Work out the finished part from the listing and answer in its coordinate system (mm). Face numbers are marked on the shaded views. A direction names the side the tool comes from. Give positions to 0.01 mm unless a question says otherwise; leave off trailing zeros. Loops run counter-clockwise (first coordinate to the right, second up) from the corner with the lowest first, then second, coordinate; pieces in that order, holes last. Notation, with made-up numbers: (0, 26.25) - (40, 26.25) arc R31 cw to (40, 55.25) - close; hole circle Ø4 at (27, -17). An arc over 180 degrees is marked (long way). One line per item, written item: value.
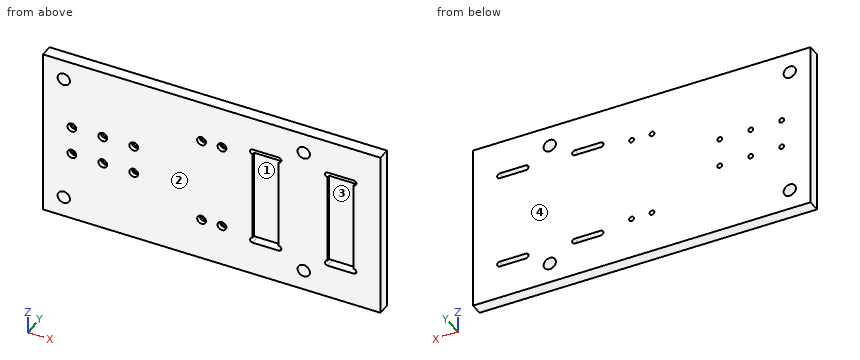
from build123d import *

# Parameters (mm, degrees)
SKETCH1_W                                      = 304.8
SKETCH1_H                                      = 152.4
BOSS_EXTRUDE1_DEPTH                            = 11.1125
CUT_EXTRUDE2_DEPTH                             = 11.1125
SKETCH10_R                                     = 5.55625
CUT_EXTRUDE9_DEPTH                             = 12.1125
CBORE_FOR_8_SOCKET_HEAD_CAP_SCREW1_D           = 4.3053
CBORE_FOR_8_SOCKET_HEAD_CAP_SCREW1_DEPTH       = 11.1125
CBORE_FOR_8_SOCKET_HEAD_CAP_SCREW1_CBORE_D     = 7.9375
CBORE_FOR_8_SOCKET_HEAD_CAP_SCREW1_CBORE_DEPTH = 4.1656
CBORE_FOR_8_SOCKET_HEAD_CAP_SCREW2_D           = 4.3053
CBORE_FOR_8_SOCKET_HEAD_CAP_SCREW2_DEPTH       = 11.1125
CBORE_FOR_8_SOCKET_HEAD_CAP_SCREW2_CBORE_D     = 7.9375
CBORE_FOR_8_SOCKET_HEAD_CAP_SCREW2_CBORE_DEPTH = 4.1656
CUT_EXTRUDE10_REACH                            = 119.196
SKETCH22_W                                     = 23.527686488
SKETCH22_H                                     = 2.54
SKETCH22_W_2                                   = 23.436556581


with BuildPart() as part:
    # Sketch1 → Boss-Extrude1 (new body)
    with BuildSketch(Plane(origin=(0, 0, 0), x_dir=(1, 0, 0), z_dir=(0, 1, 0))):
        with Locations((152.4, 76.2)):
            Rectangle(SKETCH1_W, SKETCH1_H)
    extrude(amount=BOSS_EXTRUDE1_DEPTH)

    # Sketch3 → Cut-Extrude2 (cut)
    with BuildSketch(Plane(origin=(0, 11.1125, 0), x_dir=(1, 0, 0), z_dir=(0, 1, 0))):
        with BuildLine():
            Line((280.567699438, 35.204123045), (257.04001295, 35.204123045))
            ThreePointArc((257.04001295, 35.204123045), (254.65876295, 32.822873045), (257.04001295, 30.441623045))
            Line((257.04001295, 30.441623045), (280.567699438, 30.441623045))
            ThreePointArc((280.567699438, 30.441623045), (282.948949438, 32.822873045), (280.567699438, 35.204123045))
        make_face()
        with BuildLine():
            Line((257.04001295, 117.195876955), (280.567699438, 117.195876955))
            ThreePointArc((280.567699438, 117.195876955), (282.948949438, 119.577126955), (280.567699438, 121.958376955))
            Line((280.567699438, 121.958376955), (257.04001295, 121.958376955))
            ThreePointArc((257.04001295, 121.958376955), (254.65876295, 119.577126955), (257.04001295, 117.195876955))
        make_face()
        with BuildLine():
            Line((212.85998705, 121.958376955), (189.332300562, 121.958376955))
            ThreePointArc((189.332300562, 121.958376955), (186.951050562, 119.577126955), (189.332300562, 117.195876955))
            Line((189.332300562, 117.195876955), (212.85998705, 117.195876955))
            ThreePointArc((212.85998705, 117.195876955), (215.24123705, 119.577126955), (212.85998705, 121.958376955))
        make_face()
        with BuildLine():
            Line((212.85998705, 35.204123045), (189.332300562, 35.204123045))
            ThreePointArc((189.332300562, 35.204123045), (186.951050562, 32.822873045), (189.332300562, 30.441623045))
            Line((189.332300562, 30.441623045), (212.85998705, 30.441623045))
            ThreePointArc((212.85998705, 30.441623045), (215.24123705, 32.822873045), (212.85998705, 35.204123045))
        make_face()
    extrude(amount=-CUT_EXTRUDE2_DEPTH, mode=Mode.SUBTRACT)

    # Sketch10 → Cut-Extrude9 (cut, through all)
    with BuildSketch(Plane.XZ):
        with Locations((18.74955505, -134.149424539)):
            Circle(SKETCH10_R)
        with Locations((18.74955505, -18.250575461)):
            Circle(SKETCH10_R)
        with Locations((235.448687079, -134.149424539)):
            Circle(SKETCH10_R)
        with Locations((235.448687079, -18.250575461)):
            Circle(SKETCH10_R)
    extrude(amount=-CUT_EXTRUDE9_DEPTH, mode=Mode.SUBTRACT)

    # CBORE for #8 Socket Head Cap Screw1
    with Locations(Plane(origin=(143.1925, 0, -37.545187713), x_dir=(0, 0, -1), z_dir=(0, -1, 0))):
        with Locations((0, 0), (0, 18.415), (77.309624574, 18.415), (77.309624574, 0)):
            CounterBoreHole(CBORE_FOR_8_SOCKET_HEAD_CAP_SCREW1_D / 2, CBORE_FOR_8_SOCKET_HEAD_CAP_SCREW1_CBORE_D / 2, CBORE_FOR_8_SOCKET_HEAD_CAP_SCREW1_CBORE_DEPTH, depth=CBORE_FOR_8_SOCKET_HEAD_CAP_SCREW1_DEPTH)

    # CBORE for #8 Socket Head Cap Screw2
    with Locations(Plane(origin=(26.061945565, 0, -89.133574987), x_dir=(0, 0, -1), z_dir=(0, -1, 0))):
        with Locations((0, 0), (-25.867149974, 0), (-25.867149974, 27.94), (0, 27.94), (0, 55.88), (-25.867149974, 55.88)):
            CounterBoreHole(CBORE_FOR_8_SOCKET_HEAD_CAP_SCREW2_D / 2, CBORE_FOR_8_SOCKET_HEAD_CAP_SCREW2_CBORE_D / 2, CBORE_FOR_8_SOCKET_HEAD_CAP_SCREW2_CBORE_DEPTH, depth=CBORE_FOR_8_SOCKET_HEAD_CAP_SCREW2_DEPTH)

    # Sketch22 → Cut-Extrude10 (cut, up to next)
    with BuildSketch(Plane.XY.offset(-35.204123045), mode=Mode.PRIVATE) as cut_extrude10_sk1:
        with Locations((201.096143806, 1.27)):
            Rectangle(SKETCH22_W, SKETCH22_H)
    cut_extrude10_tool1 = extrude(cut_extrude10_sk1.sketch, amount=-CUT_EXTRUDE10_REACH, mode=Mode.PRIVATE) & part.part
    add(cut_extrude10_tool1.solids().sort_by_distance((201.096144, 1.27, -35.204123))[0], mode=Mode.SUBTRACT)
    # Sketch22 → Cut-Extrude10 (cut, up to next)
    with BuildSketch(Plane.XY.offset(-35.204123045), mode=Mode.PRIVATE) as cut_extrude10_sk2:
        with Locations((268.758291241, 1.27)):
            Rectangle(SKETCH22_W_2, SKETCH22_H)
    cut_extrude10_tool2 = extrude(cut_extrude10_sk2.sketch, amount=-CUT_EXTRUDE10_REACH, mode=Mode.PRIVATE) & part.part
    add(cut_extrude10_tool2.solids().sort_by_distance((268.758291, 1.27, -35.204123))[0], mode=Mode.SUBTRACT)


solid = part.part
1. Section C-C (y = 9) is taken. Count the separate pieces of the cut face and the enclosed holes in it, and give its area (3 significant figures).
Output:
separate pieces: 1
enclosed holes: 18
area: 45,400 mm²
2. The mould has two halves that part along Z. Classify the marked faces 1 and 2: released by +Z, released by -Z, zero draft, split by the parting line, or undercut.
Output:
face 1: undercut
face 2: zero draft
3. Section A-A (x = 209.5) is taken. Write down the section's boundary in (y, z).
Output:
outline: (0, -152.4) - (11.11, -152.4) - (11.11, -121.96) - (0, -121.96) - close; (0, -30.44) - (11.11, -30.44) - (11.11, 0) - (0, 0) - close; (2.54, -117.2) - (11.11, -117.2) - (11.11, -35.2) - (2.54, -35.2) - close
4. Section B-B (z = -73.5) is taken. Write down the section's boundary in (x, y).
Output:
outline: (0, 0) - (189.33, 0) - (189.33, 2.54) - (212.86, 2.54) - (212.86, 0) - (257.04, 0) - (257.04, 2.54) - (280.48, 2.54) - (280.48, 0) - (304.8, 0) - (304.8, 11.11) - (0, 11.11) - close
5. A flat-ended cylindrical pin translates along its axis: pin 1 Ø7 at (x, z) = (143.19, -114.85) entering from -Y. Find the tip coordinate at first contact, or state that the pin passes through.
Output:
pin 1: stops at y = 4.17
6. Find the intervals of material crossed by line 1 along Z through (x, y) = (257, 4); line 2 along X through (y, z) = (8, -32.5); line 3 along X through (y, z) = (7.5, -22.5), in increasing order.
Output:
line 1: z = -152.4 to -121.96, -117.2 to -35.2, -30.44 to 0
line 2: x = 0 to 186.97, 215.22 to 254.68, 282.93 to 304.8
line 3: x = 0 to 15.17, 22.33 to 231.87, 239.03 to 304.8
7. For the marked faces 3 and 4, determine the directions among +Z, -Z, +X, -X, +Y, -Y from which every point of the face is accessible in a straight line to the end or side of a thin tool.
Output:
face 3: -Y
face 4: +Z, -Z, +X, -X, +Y
